Work out the finished part from the listing and answer in its coordinate system (mm). A direction names the side the tool comes from. Round coordinates to 2 decimals unless told otherwise and drop trailing zeros. Order: outer loops, then holes, each group sorted by start corner. A loop starts at its lowest first (then second) coordinate and runs counter-clockwise, first axis right, second up. Notation, with made-up numbers: (6.25, 18.25) - (27.25, 18.25) arc R18 ccw to (27.25, 40.25) - close; hole circle Ø7 at (-22, 0.25). An arc over 180 degrees is marked (long way). Use one line per item in the form item = value. Start each with the question number.
Q1. The part is cut by section B-B on x = -15. Determine the outline of the cut face in (y, z).
Q2. The part is cut by section C-C on x = -6. Determine the outline of the cut face in (y, z), plus the area to 3 significant figures.
Q3. The part is cut by section A-A on z = -15. Determine the outline of the cut face in (x, y).
Q4. For a pull along Z with two mould halves and no side action, classify faces 1 (the flat face through (-27, -3, -27)), 2 (the flat face through (-18, 1, 12)), 3 (the cylindrical face through (-17.32, -1.03, 7.87)) as +Z half, -Z half, draft (parallel to the pull), parting line (faces both ways), or undercut.
Q5. Given P1, Ø14, axis at x = 10, z = 7.5, coming from the +Y side; P2, Ø1.1, axis at x = 13.5, y = 0.5, coming from the +Z side; P3, Ø3, axis at x = 11.5, z = -13.5, coming from the -Y side; P4, Ø5, axis at x = 10, z = -15, coming from the +Y side, each flat-ended and moving along its own axis, determine where each tip first touches the part or whether it passes through.
Q6. Find the intervals of material crossed by line 1 (Y direction, x = -1, z = -26); line 2 (Z direction, x = -15, y = -4.65); line 3 (Y direction, x = -4, z = 14), in increasing order. Write a range as [from, to].
Q7. The part is cut by section D-D on z = 11.5. Determine the outline of the cut face in (x, y), plus the area to 3 significant figures.
Q8. Which of the six approach directions +Z, -Z, +X, -X, +Y, -Y give full straight-line access (tool end or side, diameter ignored) to faces 4 (the flat face through (6, -2, -7.5)), 5 (the cylindrical face through (-21.494, -4.521, 9.714)), 6 (the flat face through (20, -3, -16))?
from build123d import *

# Parameters (mm, degrees)
BOX003_W          = 28
BOX003_H          = 16
BOX003_DEPTH      = 28
CYLINDER002_R     = 6.5
CYLINDER002_DEPTH = 10
CYLINDER003_R     = 6.5
CYLINDER003_DEPTH = 10
CYLINDER001_R     = 3.15
CYLINDER001_DEPTH = 10
CYLINDER_R        = 3.15
CYLINDER_DEPTH    = 10
BOX001_W          = 7.8
BOX001_H          = 2
BOX001_DEPTH      = 20
CHAMFER003_SIZE   = 1
BOX002_W          = 20
BOX002_H          = 2
BOX002_DEPTH      = 7.8
CHAMFER004_SIZE   = 1
BOX_W             = 48
BOX_H             = 6
BOX_DEPTH         = 48
CHAMFER_SIZE      = 20
CHAMFER001_SIZE   = 2
CHAMFER002_SIZE   = 1


with BuildPart() as cube003:
    # Box003 → Box003 (new body)
    with BuildSketch(Plane(origin=(-7.5, -3.5, -7.5), x_dir=(1, 0, 0), z_dir=(0, 0, 1))):
        with Locations((14, 8)):
            Rectangle(BOX003_W, BOX003_H)
    extrude(amount=BOX003_DEPTH)


with BuildPart() as cylinder002:
    # Cylinder002 → Cylinder002 (new body)
    with BuildSketch(Plane(origin=(10, -16, -15), x_dir=(1, 0, 0), z_dir=(0, 1, 0))):
        Circle(CYLINDER002_R)
    extrude(amount=CYLINDER002_DEPTH)


with BuildPart() as fusion003:
    # Cylinder003 → Cylinder003 (new body)
    with BuildSketch(Plane(origin=(-15, -16, 10), x_dir=(1, 0, 0), z_dir=(0, 1, 0))):
        Circle(CYLINDER003_R)
    extrude(amount=CYLINDER003_DEPTH)

    # Fusion003: union Cylinder002
    add(cylinder002.part)


with BuildPart() as fusion003_1:
    # Fusion003 placement: moved
    add(fusion003.part.moved(Location((0, 3, 0))))


with BuildPart() as cylinder001:
    # Cylinder001 → Cylinder001 (new body)
    with BuildSketch(Plane(origin=(10, -7, -15), x_dir=(1, 0, 0), z_dir=(0, 1, 0))):
        Circle(CYLINDER001_R)
    extrude(amount=CYLINDER001_DEPTH)


with BuildPart() as fusion002:
    # Cylinder → Cylinder (new body)
    with BuildSketch(Plane(origin=(-15, -7, 10), x_dir=(1, 0, 0), z_dir=(0, 1, 0))):
        Circle(CYLINDER_R)
    extrude(amount=CYLINDER_DEPTH)

    # Fusion002: union Cylinder001
    add(cylinder001.part)


with BuildPart() as chamfer003:
    # Box001 → Box001 (new body)
    with BuildSketch(Plane(origin=(-18.9, -1, 0), x_dir=(1, 0, 0), z_dir=(0, 0, 1))):
        with Locations((3.9, 1)):
            Rectangle(BOX001_W, BOX001_H)
    extrude(amount=BOX001_DEPTH)

    # Chamfer003
    chamfer003_edges = [chamfer003.edges().sort_by_distance(p)[0] for p in [
        (-15, 1, 0),
        (-15, 1, 20),
    ]]
    chamfer(chamfer003_edges, length=CHAMFER003_SIZE)


with BuildPart() as fusion:
    # Box002 → Box002 (new body)
    with BuildSketch(Plane(origin=(0, -1, -18.9), x_dir=(1, 0, 0), z_dir=(0, 0, 1))):
        with Locations((10, 1)):
            Rectangle(BOX002_W, BOX002_H)
    extrude(amount=BOX002_DEPTH)

    # Chamfer004
    chamfer004_edges = [fusion.edges().sort_by_distance(p)[0] for p in [
        (0, 1, -15),
        (20, 1, -15),
    ]]
    chamfer(chamfer004_edges, length=CHAMFER004_SIZE)

    # Fusion: union Chamfer003
    add(chamfer003.part)


with BuildPart() as side_corner_panel_clip:
    # Box → Box (new body)
    with BuildSketch(Plane(origin=(-28, -6, -28), x_dir=(1, 0, 0), z_dir=(0, 0, 1))):
        with Locations((24, 3)):
            Rectangle(BOX_W, BOX_H)
    extrude(amount=BOX_DEPTH)

    # Chamfer
    chamfer_edges = [side_corner_panel_clip.edges().sort_by_distance(p)[0] for p in [
        (20, -3, 20),
    ]]
    chamfer(chamfer_edges, length=CHAMFER_SIZE)

    # Chamfer001
    chamfer001_edges = [side_corner_panel_clip.edges().sort_by_distance(p)[0] for p in [
        (20, -3, -28),
        (-28, -3, -28),
        (-28, -3, 20),
    ]]
    chamfer(chamfer001_edges, length=CHAMFER001_SIZE)

    # Chamfer002
    chamfer002_edges = [side_corner_panel_clip.edges().sort_by_distance(p)[0] for p in [
        (20, -6, -13),
        (19, -6, -27),
        (10, -6, 10),
        (-4, -6, -28),
        (-13, -6, 20),
        (-27, -6, -27),
        (-27, -6, 19),
        (-28, -6, -4),
    ]]
    chamfer(chamfer002_edges, length=CHAMFER002_SIZE)

    # Fusion001: union Fusion
    add(fusion.part)

    # Cut: cut Fusion002
    add(fusion002.part, mode=Mode.SUBTRACT)

    # Cut001: cut Fusion003
    add(fusion003_1.part, mode=Mode.SUBTRACT)

    # Cut002008006: cut Cube003
    add(cube003.part, mode=Mode.SUBTRACT)


solid = side_corner_panel_clip.part
Found:
q1.outline = (-6, -27) - (-5, -28) - (0, -28) - (0, 0) - (1, 1) - (1, 6.85) - (-3, 6.85) - (-3, 3.5) - (-6, 3.5) - close; (-6, 16.5) - (-3, 16.5) - (-3, 13.15) - (1, 13.15) - (1, 19) - (0, 20) - (-5, 20) - (-6, 19) - close
q2.outline = (-6, -27) - (-5, -28) - (0, -28) - (0, -7.5) - (-3.5, -7.5) - (-3.5, 20) - (-5, 20) - (-6, 19) - close
q2.area = 191 mm²
q3.outline = (-28, -5) - (-27, -6) - (3.5, -6) - (3.5, -3) - (6.85, -3) - (6.85, 1) - (1, 1) - (0, 0) - (-28, 0) - close; (13.15, -3) - (16.5, -3) - (16.5, -6) - (19, -6) - (20, -5) - (20, 0) - (19, 1) - (13.15, 1) - close
q4.face_1 = -Z half
q4.face_2 = draft
q4.face_3 = undercut
q5.P1 = -3.5
q5.P2 = -7.5
q5.P3 = -3
q5.P4 = through
q6.line_1 = [-6, 0]
q6.line_2 = [-28, 3.5], [16.5, 20]
q6.line_3 = [-6, -3.5]
q7.outline = (-28, -5) - (-27, -6) - (-21.32, -6) - (-21.32, -3) - (-17.77, -3) - (-17.77, 1) - (-18.9, 1) - (-18.9, 0) - (-28, 0) - close; (-12.23, -3) - (-8.68, -3) - (-8.68, -6) - (7.09, -6) - (8.5, -5) - (8.5, -3.5) - (-7.5, -3.5) - (-7.5, 0) - (-11.1, 0) - (-11.1, 1) - (-12.23, 1) - close
q7.area = 109 mm²
q8.face_4 = +Z, +X, +Y
q8.face_5 = -Y
q8.face_6 = +Z, -Z, +X, +Y, -Y
